Source: CAD feature listing. Evaluate the final solid. Frame: model axes, mm. Give positions to 0.01 mm unless a question says otherwise; leave off trailing zeros. Loops run counter-clockwise (first coordinate to the right, second up) from the corner with the lowest first, then second, coordinate; pieces in that order, holes last. Notation, with made-up numbers: (-28, 20.5) -> (-15, 20.5) arc R34 cw to (-15, 51.5) -> close; hole circle Ø9 at (15, 36.5). An arc over 180 degrees is marked (long way). Answer as a JSON object with one key per item and string values. Group by question number.
from build123d import *

# Parameters (mm, degrees)
BOSS_EXTRUDE1_DEPTH = 5
CUT_EXTRUDE1_REACH  = 64.682
SKETCH2_R           = 2
CUT_EXTRUDE2_REACH  = 64.682
SKETCH3_R           = 2


with BuildPart() as part:
    # Sketch1 → Boss-Extrude1 (new body)
    with BuildSketch(Plane(origin=(0, 0, 0), x_dir=(1, 0, 0), z_dir=(0, 1, 0))):
        with BuildLine():
            Line((40, 48), (-40, 48))
            Line((-40, 48), (-13.039417607, 0.585582393))
            ThreePointArc((-13.039417607, 0.585582393), (0, -7), (13.039417607, 0.585582393))
            Line((13.039417607, 0.585582393), (40, 48))
        make_face()
    extrude(amount=BOSS_EXTRUDE1_DEPTH)

    # Sketch2 → Cut-Extrude1 (cut, up to next)
    with BuildSketch(Plane(origin=(0, 5, 0), x_dir=(1, 0, 0), z_dir=(0, 1, 0)), mode=Mode.PRIVATE) as cut_extrude1_sk1:
        with Locations(Location((-25, 35, 0), (0, 0, 270))):
            Circle(SKETCH2_R)
    cut_extrude1_tool1 = extrude(cut_extrude1_sk1.sketch, amount=-CUT_EXTRUDE1_REACH, mode=Mode.PRIVATE) & part.part
    cut_extrude1 = cut_extrude1_tool1.solids().sort_by_distance((-25, 5, -35))[0]
    add(cut_extrude1, mode=Mode.SUBTRACT)

    # Mirror1: Cut-Extrude1 across plane
    add(cut_extrude1.mirror(Plane(origin=(0, 0, 0), x_dir=(0, 0, 1), z_dir=(1, 0, 0))), mode=Mode.SUBTRACT)

    # Sketch3 → Cut-Extrude2 (cut, up to next)
    with BuildSketch(Plane(origin=(0, 5, 0), x_dir=(1, 0, 0), z_dir=(0, 1, 0)), mode=Mode.PRIVATE) as cut_extrude2_sk1:
        with Locations(Location((0, 0, 0), (0, 0, 270))):
            Circle(SKETCH3_R)
    cut_extrude2_tool1 = extrude(cut_extrude2_sk1.sketch, amount=-CUT_EXTRUDE2_REACH, mode=Mode.PRIVATE) & part.part
    add(cut_extrude2_tool1.solids().sort_by_distance((0, 5, 0))[0], mode=Mode.SUBTRACT)


solid = part.part
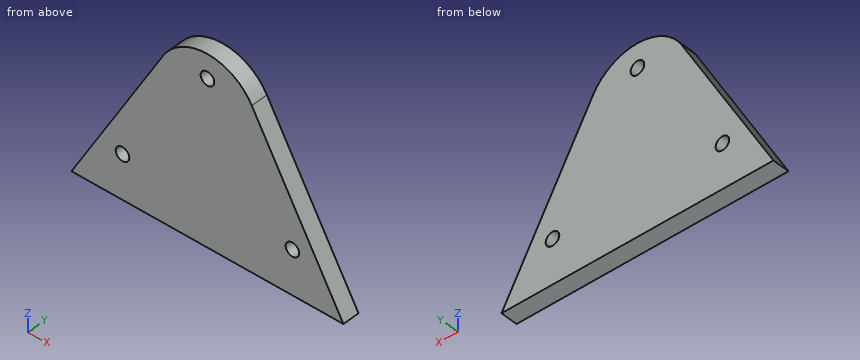
(1) Section query B-B on x = 0. Return the cut outline in (y, z).
(2) First-contact query: pin 1 (3 mm diameter, centred on x = -29, y = 1, fed in from +Z); pin 2 (3 mm diameter, centred on x = -4, y = 1, fed in from +Z); pin 3 (5 mm diameter, centred on x = 0, z = 0, fed in from -Y). Flat tips, straight axial feed; report the tip coordinate or a pass-through.
(3) Section query D-D on x = 26. Return the cut outline in (y, z), plus the area to 3 significant figures.
(4) Section query C-C on z = -35. Return the cut outline in (x, y).
(5) Section query A-A on y = 1.8. Return the cut outline in (x, z).
(6) Material intervals for line 1 (X direction, y = 2.2, z = -35); line 2 (X direction, y = 2.75, z = 0); line 3 (Z direction, x = -26.5, y = 2.5), sorted ascending. Write a range as from..to.
Result:
{
 "1": {"outline": "(0, -48) -> (5, -48) -> (5, -2) -> (0, -2) -> close; (0, 2) -> (5, 2) -> (5, 7) -> (0, 7) -> close"},
 "2": {"pin 1": "z = -26.02", "pin 2": "z = 6.79", "pin 3": "y = 0"},
 "3": {"outline": "(0, -48) -> (5, -48) -> (5, -36.73) -> (0, -36.73) -> close; (0, -33.27) -> (5, -33.27) -> (5, -23.38) -> (0, -23.38) -> close", "area": "106 mm²"},
 "4": {"outline": "(-32.61, 0) -> (-27, 0) -> (-27, 5) -> (-32.61, 5) -> close; (-23, 0) -> (23, 0) -> (23, 5) -> (-23, 5) -> close; (27, 0) -> (32.61, 0) -> (32.61, 5) -> (27, 5) -> close"},
 "5": {"outline": "(-40, -48) -> (40, -48) -> (13.04, -0.59) arc R15 ccw to (-13.04, -0.59) -> close; hole circle Ø4 at (-25, -35); hole circle Ø4 at (0, 0); hole circle Ø4 at (25, -35)"},
 "6": {"line 1": "-32.61..-27, -23..23, 27..32.61", "line 2": "-12.69..-2, 2..12.69", "line 3": "-48..-36.32, -33.68..-24.26"}
}
